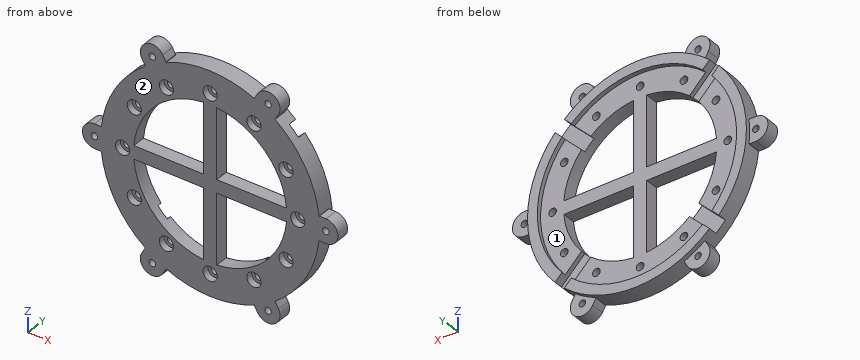
```python
from build123d import *

# Parameters (mm, degrees)
SKETCH1_R           = 50
BOSS_EXTRUDE1_DEPTH = 8
SKETCH2_R           = 45.5
CUT_EXTRUDE1_DEPTH  = 2
SKETCH3_R           = 1.75
CUT_EXTRUDE2_DEPTH  = 72.161787499
SKETCH4_R           = 3.25
CUT_EXTRUDE3_DEPTH  = 3
BOSS_EXTRUDE2_DEPTH = 6
SKETCH6_R           = 1.5
CUT_EXTRUDE4_DEPTH  = 79.087932515
CUT_EXTRUDE6_DEPTH  = 78.908441164
CUT_EXTRUDE9_DEPTH  = 4


with BuildPart() as part:
    # Sketch1 → Boss-Extrude1 (new body)
    with BuildSketch(Plane(origin=(0, 0, 0), x_dir=(1, 0, 0), z_dir=(0, 1, 0))):
        with Locations(Location((0, 0, 0), (0, 0, 270))):
            Circle(SKETCH1_R)
    extrude(amount=BOSS_EXTRUDE1_DEPTH)

    # Sketch2 → Cut-Extrude1 (cut)
    with BuildSketch(Plane(origin=(0, 8, 0), x_dir=(1, 0, 0), z_dir=(0, 1, 0))):
        with Locations(Location((0, 0, 0), (0, 0, 270))):
            Circle(SKETCH2_R)
    extrude(amount=-CUT_EXTRUDE1_DEPTH, mode=Mode.SUBTRACT)

    # Sketch3 → Cut-Extrude2 (cut, through all)
    with BuildSketch(Plane.XZ):
        with Locations(Location((-40, 0, 0), (0, 0, 270))):
            Circle(SKETCH3_R)
        with Locations(Location((-34.641016151, 20, 0), (0, 0, 270))):
            Circle(SKETCH3_R)
        with Locations(Location((-20, 34.641016151, 0), (0, 0, 270))):
            Circle(SKETCH3_R)
        with Locations(Location((0, 40, 0), (0, 0, 270))):
            Circle(SKETCH3_R)
        with Locations(Location((20, 34.641016151, 0), (0, 0, 270))):
            Circle(SKETCH3_R)
        with Locations(Location((34.641016151, 20, 0), (0, 0, 270))):
            Circle(SKETCH3_R)
        with Locations(Location((40, 0, 0), (0, 0, 270))):
            Circle(SKETCH3_R)
        with Locations(Location((34.641016151, -20, 0), (0, 0, 270))):
            Circle(SKETCH3_R)
        with Locations(Location((20, -34.641016151, 0), (0, 0, 270))):
            Circle(SKETCH3_R)
        with Locations(Location((0, -40, 0), (0, 0, 270))):
            Circle(SKETCH3_R)
        with Locations(Location((-20, -34.641016151, 0), (0, 0, 270))):
            Circle(SKETCH3_R)
        with Locations(Location((-34.641016151, -20, 0), (0, 0, 270))):
            Circle(SKETCH3_R)
    extrude(amount=-CUT_EXTRUDE2_DEPTH, mode=Mode.SUBTRACT)

    # Sketch4 → Cut-Extrude3 (cut)
    with BuildSketch(Plane.XZ):
        with Locations(Location((-40, 0, 0), (0, 0, 270))):
            Circle(SKETCH4_R)
        with Locations(Location((-34.641016151, 20, 0), (0, 0, 270))):
            Circle(SKETCH4_R)
        with Locations(Location((-20, 34.641016151, 0), (0, 0, 270))):
            Circle(SKETCH4_R)
        with Locations(Location((0, 40, 0), (0, 0, 270))):
            Circle(SKETCH4_R)
        with Locations(Location((20, 34.641016151, 0), (0, 0, 270))):
            Circle(SKETCH4_R)
        with Locations(Location((34.641016151, 20, 0), (0, 0, 270))):
            Circle(SKETCH4_R)
        with Locations(Location((40, 0, 0), (0, 0, 270))):
            Circle(SKETCH4_R)
        with Locations(Location((34.641016151, -20, 0), (0, 0, 270))):
            Circle(SKETCH4_R)
        with Locations(Location((20, -34.641016151, 0), (0, 0, 270))):
            Circle(SKETCH4_R)
        with Locations(Location((0, -40, 0), (0, 0, 270))):
            Circle(SKETCH4_R)
        with Locations(Location((-20, -34.641016151, 0), (0, 0, 270))):
            Circle(SKETCH4_R)
        with Locations(Location((-34.641016151, -20, 0), (0, 0, 270))):
            Circle(SKETCH4_R)
    extrude(amount=-CUT_EXTRUDE3_DEPTH, mode=Mode.SUBTRACT)

    # Sketch5 → Boss-Extrude2 (add)
    with BuildSketch(Plane.XZ):
        with BuildLine():
            Line((50, 5.481362668), (52.872058145, 5.481362668))
            ThreePointArc((52.872058145, 5.481362668), (58.353420813, 0), (52.872058145, -5.481362668))
            Line((52.872058145, -5.481362668), (50, -5.481362668))
            ThreePointArc((50, -5.481362668), (49.849716822, -5.479302115), (49.699546633, -5.473122004))
            ThreePointArc((49.699546633, -5.473122004), (50, 0), (49.699546633, 5.473122004))
            ThreePointArc((49.699546633, 5.473122004), (49.849716822, 5.479302115), (50, 5.481362668))
        make_face()
        with BuildLine():
            Line((29.746999318, -40.560588855), (31.18302839, -43.04786417))
            ThreePointArc((31.18302839, -43.04786417), (29.176710406, -50.535544822), (21.689029755, -48.529226838))
            Line((21.689029755, -48.529226838), (20.253000682, -46.041951523))
            ThreePointArc((20.253000682, -46.041951523), (20.179643585, -45.910772197), (20.109910623, -45.777630943))
            ThreePointArc((20.109910623, -45.777630943), (25, -43.301270189), (29.58963601, -40.304508939))
            ThreePointArc((29.58963601, -40.304508939), (29.670073237, -40.431470082), (29.746999318, -40.560588855))
        make_face()
        with BuildLine():
            Line((-20.253000682, -46.041951523), (-21.689029755, -48.529226838))
            ThreePointArc((-21.689029755, -48.529226838), (-29.176710406, -50.535544822), (-31.18302839, -43.04786417))
            Line((-31.18302839, -43.04786417), (-29.746999318, -40.560588855))
            ThreePointArc((-29.746999318, -40.560588855), (-29.670073237, -40.431470082), (-29.58963601, -40.304508939))
            ThreePointArc((-29.58963601, -40.304508939), (-25, -43.301270189), (-20.109910623, -45.777630943))
            ThreePointArc((-20.109910623, -45.777630943), (-20.179643585, -45.910772197), (-20.253000682, -46.041951523))
        make_face()
        with BuildLine():
            Line((-50, -5.481362668), (-52.872058145, -5.481362668))
            ThreePointArc((-52.872058145, -5.481362668), (-58.353420813, 0), (-52.872058145, 5.481362668))
            Line((-52.872058145, 5.481362668), (-50, 5.481362668))
            ThreePointArc((-50, 5.481362668), (-49.849716822, 5.479302115), (-49.699546633, 5.473122004))
            ThreePointArc((-49.699546633, 5.473122004), (-50, 0), (-49.699546633, -5.473122004))
            ThreePointArc((-49.699546633, -5.473122004), (-49.849716822, -5.479302115), (-50, -5.481362668))
        make_face()
        with BuildLine():
            Line((-29.746999318, 40.560588855), (-31.18302839, 43.04786417))
            ThreePointArc((-31.18302839, 43.04786417), (-29.176710406, 50.535544822), (-21.689029755, 48.529226838))
            Line((-21.689029755, 48.529226838), (-20.253000682, 46.041951523))
            ThreePointArc((-20.253000682, 46.041951523), (-20.179643585, 45.910772197), (-20.109910623, 45.777630943))
            ThreePointArc((-20.109910623, 45.777630943), (-25, 43.301270189), (-29.58963601, 40.304508939))
            ThreePointArc((-29.58963601, 40.304508939), (-29.670073237, 40.431470082), (-29.746999318, 40.560588855))
        make_face()
        with BuildLine():
            Line((20.253000682, 46.041951523), (21.689029755, 48.529226838))
            ThreePointArc((21.689029755, 48.529226838), (29.176710406, 50.535544822), (31.18302839, 43.04786417))
            Line((31.18302839, 43.04786417), (29.746999318, 40.560588855))
            ThreePointArc((29.746999318, 40.560588855), (29.670073237, 40.431470082), (29.58963601, 40.304508939))
            ThreePointArc((29.58963601, 40.304508939), (25, 43.301270189), (20.109910623, 45.777630943))
            ThreePointArc((20.109910623, 45.777630943), (20.179643585, 45.910772197), (20.253000682, 46.041951523))
        make_face()
    extrude(amount=-BOSS_EXTRUDE2_DEPTH)

    # Sketch6 → Cut-Extrude4 (cut, through all)
    with BuildSketch(Plane.XZ):
        with Locations(Location((52.872058145, 0, 0), (0, 0, 270))):
            Circle(SKETCH6_R)
        with Locations(Location((26.436029072, -45.788545504, 0), (0, 0, 270))):
            Circle(SKETCH6_R)
        with Locations(Location((-26.436029072, -45.788545504, 0), (0, 0, 270))):
            Circle(SKETCH6_R)
        with Locations(Location((-52.872058145, 0, 0), (0, 0, 270))):
            Circle(SKETCH6_R)
        with Locations(Location((-26.436029072, 45.788545504, 0), (0, 0, 270))):
            Circle(SKETCH6_R)
        with Locations(Location((26.436029072, 45.788545504, 0), (0, 0, 270))):
            Circle(SKETCH6_R)
    extrude(amount=-CUT_EXTRUDE4_DEPTH, mode=Mode.SUBTRACT)

    # Sketch9 → Cut-Extrude6 (cut, through all)
    with BuildSketch(Plane(origin=(0, 6, 0), x_dir=(1, 0, 0), z_dir=(0, 1, 0))):
        with BuildLine():
            Line((-3, -3), (-3, -34.871191548))
            ThreePointArc((-3, -34.871191548), (-24.748737342, -24.748737342), (-34.871191548, -3))
            Line((-34.871191548, -3), (-3, -3))
        make_face()
        with BuildLine():
            Line((-3, 3), (-34.871191548, 3))
            ThreePointArc((-34.871191548, 3), (-24.748737342, 24.748737342), (-3, 34.871191548))
            Line((-3, 34.871191548), (-3, 3))
        make_face()
        with BuildLine():
            Line((3, 3), (3, 34.871191548))
            ThreePointArc((3, 34.871191548), (24.748737342, 24.748737342), (34.871191548, 3))
            Line((34.871191548, 3), (3, 3))
        make_face()
        with BuildLine():
            Line((3, -3), (34.871191548, -3))
            ThreePointArc((34.871191548, -3), (24.748737342, -24.748737342), (3, -34.871191548))
            Line((3, -34.871191548), (3, -3))
        make_face()
    extrude(amount=-CUT_EXTRUDE6_DEPTH, mode=Mode.SUBTRACT)

    # Sketch10 → Cut-Extrude9 (cut)
    with BuildSketch(Plane(origin=(0, 8, 0), x_dir=(1, 0, 0), z_dir=(0, 1, 0))):
        with BuildLine():
            Line((-24.054791846, 19.812151159), (-37.476659403, 33.234018716))
            ThreePointArc((-37.476659403, 33.234018716), (-37.476659403, 37.476659403), (-33.234018716, 37.476659403))
            Line((-33.234018716, 37.476659403), (-19.812151159, 24.054791846))
            ThreePointArc((-19.812151159, 24.054791846), (-22.035815668, 22.035815668), (-24.054791846, 19.812151159))
        make_face()
        with BuildLine():
            Line((19.812151159, 24.054791846), (33.234018716, 37.476659403))
            ThreePointArc((33.234018716, 37.476659403), (37.476659403, 37.476659403), (37.476659403, 33.234018716))
            Line((37.476659403, 33.234018716), (24.054791846, 19.812151159))
            ThreePointArc((24.054791846, 19.812151159), (22.035815668, 22.035815668), (19.812151159, 24.054791846))
        make_face()
        with BuildLine():
            Line((24.054791846, -19.812151159), (37.476659403, -33.234018716))
            ThreePointArc((37.476659403, -33.234018716), (37.476659403, -37.476659403), (33.234018716, -37.476659403))
            Line((33.234018716, -37.476659403), (19.812151159, -24.054791846))
            ThreePointArc((19.812151159, -24.054791846), (22.035815668, -22.035815668), (24.054791846, -19.812151159))
        make_face()
        with BuildLine():
            Line((-19.812151159, -24.054791846), (-33.234018716, -37.476659403))
            ThreePointArc((-33.234018716, -37.476659403), (-37.476659403, -37.476659403), (-37.476659403, -33.234018716))
            Line((-37.476659403, -33.234018716), (-24.054791846, -19.812151159))
            ThreePointArc((-24.054791846, -19.812151159), (-22.035815668, -22.035815668), (-19.812151159, -24.054791846))
        make_face()
    extrude(amount=-CUT_EXTRUDE9_DEPTH, mode=Mode.SUBTRACT)


solid = part.part
```
Geometry check sheet. Reference: the model listing, model coordinates, mm. Face numbers are marked on the shaded views. Round coordinates to 2 decimals unless told otherwise and drop trailing zeros. Loops run counter-clockwise (first coordinate to the right, second up) from the corner with the lowest first, then second, coordinate; pieces in that order, holes last. Notation, with made-up numbers: (-36, -8.5) - (-2, -8.5) arc R15 cw to (-2, 10.5) - close; hole circle Ø6 at (78.5, -3). An arc over 180 degrees is marked (long way). Write item = value, one per line. Start each with the question number.
1. Depth check by flat-ended pin: pin 1 (7 mm diameter, centred on x = 0, z = 40, fed in from -Y); pin 2 (2 mm diameter, centred on y = 7, z = 31, fed in from -X); pin 3 (2 mm diameter, centred on y = 4, z = 27, fed in from -X); pin 4 (3 mm diameter, centred on y = 2.5, z = -6.5, fed in from +X). Enter the tip coordinate at first touch or a pass-through.
2. Section check D-D on z = -13.5. Enter the section's corners in (x, y).
3. Section check A-A on x = 0. Enter the section's corners in (y, z), then the cut area to 3 significant figures.
4. Thickness scan on line 1 (X direction, y = 4, z = -12); line 2 (Z direction, x = -26.5, y = 5.75); line 3 (Z direction, x = 1, y = 6.5). Record the ranges inside material, lowest first.
5. Section check B-B on z = 20. Give the number of separate pieces and of enclosed holes in the cut face, then the cut area to 3 significant figures.
6. Section check C-C on x = -40. Enter the section's corners in (y, z).
7. Mould release check, pull along Z, two halves, no side actions. Record for the marked faces 1 and 2: released by +Z, released by -Z, zero draft, split by the parting line, or undercut.
Working result:
q1.pin_1 = 0
q1.pin_2 = -40
q1.pin_3 = -42.71
q1.pin_4 = 55.12
q2.outline = (-48.14, 0) - (-32.29, 0) - (-32.29, 6) - (-43.45, 6) - (-43.45, 8) - (-48.14, 8) - close; (-3, 0) - (3, 0) - (3, 6) - (-3, 6) - close; (32.29, 0) - (48.14, 0) - (48.14, 8) - (43.45, 8) - (43.45, 6) - (32.29, 6) - close
q3.outline = (0, -50) - (8, -50) - (8, -45.5) - (6, -45.5) - (6, -41.75) - (3, -41.75) - (3, -43.25) - (0, -43.25) - close; (0, -36.75) - (3, -36.75) - (3, -38.25) - (6, -38.25) - (6, 38.25) - (3, 38.25) - (3, 36.75) - (0, 36.75) - close; (0, 43.25) - (3, 43.25) - (3, 41.75) - (6, 41.75) - (6, 45.5) - (8, 45.5) - (8, 50) - (0, 50) - close
q3.area = 558 mm^2
q4.line_1 = -48.54 to -32.88, -3 to 3, 32.88 to 48.54
q4.line_2 = -51.27 to -47.29, -44.29 to -30.74, -3 to 3, 30.74 to 44.29, 47.29 to 51.27
q4.line_3 = -49.99 to -45.49, 45.49 to 49.99
q5.separate_pieces = 5
q5.enclosed_holes = 0
q5.area = 201 mm^2
q6.outline = (0, -30) - (8, -30) - (8, -21.69) - (6, -21.69) - (6, -1.75) - (3, -1.75) - (3, -3.25) - (0, -3.25) - close; (0, 3.25) - (3, 3.25) - (3, 1.75) - (6, 1.75) - (6, 21.69) - (8, 21.69) - (8, 30) - (0, 30) - close
q7.face_1 = undercut
q7.face_2 = zero draft
